Read the model definition and answer for the solid it produces. Units are mm, in the model's axes. A direction names the side the tool comes from. Coordinates: 2 decimals unless noted, no trailing zeros. Loops run counter-clockwise (first coordinate to the right, second up) from the corner with the lowest first, then second, coordinate; pieces in that order, holes last. Notation, with made-up numbers: (43, 57.5) -> (95, 57.5) arc R15 ccw to (95, 70.5) -> close; hole circle Ø8 at (77.25, 39.25). An arc over 180 degrees is marked (long way). Answer as a JSON object with one key per item and string values. Group by question number.
1) Section D-D, the plane y = 33.5 is taken. Give the vertices of the cut face in (x, z).
2) Section A-A, the plane x = -49 is taken. Give the vertices of the cut face in (y, z).
3) Flat-ended cylindrical pins translate along their axes: P1, Ø4, axis at y = 41, z = 36, coming from the -X side; P2, Ø16, axis at x = -5.5, z = 12.5, coming from the +Y side; P3, Ø3, axis at y = 46, z = 19, coming from the +X side. Find the tip coordinate at first contact, or state that the pin passes through.
4) Section B-B, the plane y = 26 is taken. Give the vertices of the cut face in (x, z), plus the area to 3 significant figures.
5) Determine the mould class of faces 1 (the face through (-33.558, 24, 20)), 2 (the face through (-13.558, 24, 20)), 3 (the face through (-3.558, 28, 20)), 4 (the face through (-24, 34, 0)) for opening direction X: released by +X, released by -X, zero draft, split by the parting line, or undercut.
6) Which of the six approach directions +Z, -Z, +X, -X, +Y, -Y give full straight-line access (tool end or side, diameter ignored) to faces 5 (the face through (-49, 28, 30)), 6 (the face through (-41, 38.633, 20)), 7 (the face through (-6, 38.633, 20)), 8 (the face through (1, 28, 30)), 9 (the face through (-53.558, 29, 35))?
7) Section C-C, the plane z = 13 is taken. Give the vertices of the cut face in (x, y).
8) Consider probe 1 along Z at (x, y) = (-3.5, 22.25); probe 2 along X at (y, z) = (23.25, 25); probe 3 along Y at (x, z) = (-36.5, 12). Determine where each line is inside the solid, lowest interval first. Write a range as [from, to].
from build123d import *

# Parameters (mm, degrees)
F1_DEPTH = 40
F2_W     = 10
F2_H     = 20
F3_DEPTH = 30.001
F4_W     = 10
F4_H     = 20
F5_DEPTH = 30.001


with BuildPart() as f1:
    # F0 (on Top) → F1 (new body)
    with BuildSketch(Plane.XY):
        Polygon((-33.55762, 38.633292), (-53.55762, 38.633292), (-53.55762, 18.633292), (-33.55762, 18.633292), (-33.55762, 28.633292), (-13.55762, 28.633292), (-13.55762, 18.633292), (6.44238, 18.633292), (6.44238, 38.633292), (-13.55762, 38.633292), (-13.55762, 48.633292), (-33.55762, 48.633292), align=None)
    extrude(amount=F1_DEPTH)

    # F2 (on face) → F3 (cut, through all)
    with BuildSketch(Plane.XZ.offset(-18.633292)):
        with Locations((-48.55762, 20)):
            Rectangle(F2_W, F2_H)
    extrude(amount=-F3_DEPTH, mode=Mode.SUBTRACT)

    # F4 (on face) → F5 (cut, through all)
    with BuildSketch(Plane.XZ.offset(-18.633292)):
        with Locations((1.44238, 20)):
            Rectangle(F4_W, F4_H)
    extrude(amount=-F5_DEPTH, mode=Mode.SUBTRACT)


solid = f1.part
Determined:
{
 "1": {"outline": "(-53.56, 0) -> (6.44, 0) -> (6.44, 10) -> (-3.56, 10) -> (-3.56, 30) -> (6.44, 30) -> (6.44, 40) -> (-53.56, 40) -> (-53.56, 30) -> (-43.56, 30) -> (-43.56, 10) -> (-53.56, 10) -> close"},
 "2": {"outline": "(18.63, 0) -> (38.63, 0) -> (38.63, 10) -> (18.63, 10) -> close; (18.63, 30) -> (38.63, 30) -> (38.63, 40) -> (18.63, 40) -> close"},
 "3": {"P1": "x = -33.56", "P2": "y = 38.63", "P3": "x = -13.56"},
 "4": {"outline": "(-53.56, 0) -> (-33.56, 0) -> (-33.56, 40) -> (-53.56, 40) -> (-53.56, 30) -> (-43.56, 30) -> (-43.56, 10) -> (-53.56, 10) -> close; (-13.56, 0) -> (6.44, 0) -> (6.44, 10) -> (-3.56, 10) -> (-3.56, 30) -> (6.44, 30) -> (6.44, 40) -> (-13.56, 40) -> close", "area": "1,200 mm²"},
 "5": {"face 1": "undercut", "face 2": "undercut", "face 3": "released by +X", "face 4": "zero draft"},
 "6": {"face 5": "-X, +Y, -Y", "face 6": "+Z, -Z, -X, +Y", "face 7": "+Z, -Z, +X, +Y", "face 8": "+X, +Y, -Y", "face 9": "+Z, -Z, -X, +Y, -Y"},
 "7": {"outline": "(-43.56, 18.63) -> (-33.56, 18.63) -> (-33.56, 28.63) -> (-13.56, 28.63) -> (-13.56, 18.63) -> (-3.56, 18.63) -> (-3.56, 38.63) -> (-13.56, 38.63) -> (-13.56, 48.63) -> (-33.56, 48.63) -> (-33.56, 38.63) -> (-43.56, 38.63) -> close"},
 "8": {"probe 1": "[0, 10], [30, 40]", "probe 2": "[-43.56, -33.56], [-13.56, -3.56]", "probe 3": "[18.63, 38.63]"}
}
